Verification items for this drawing (mm, ordinates from the low corner). A direction names the side the tool comes from. Round coordinates to 2 decimals unless told otherwise and drop trailing zeros. Write each loop counter-clockwise with the first axis right and the second up, starting at its lowest first coordinate (ties: lowest second). Pieces come first, ordered by that corner, then holes. Notation, with made-up numbers: (-39, -31.5) -> (-17, -31.5) arc R27 ccw to (-17, -6.5) -> close; hole circle Ø2 at (64, 57.5). An arc over 180 degrees is marked (long way). One line per question, with ' | ' between items.
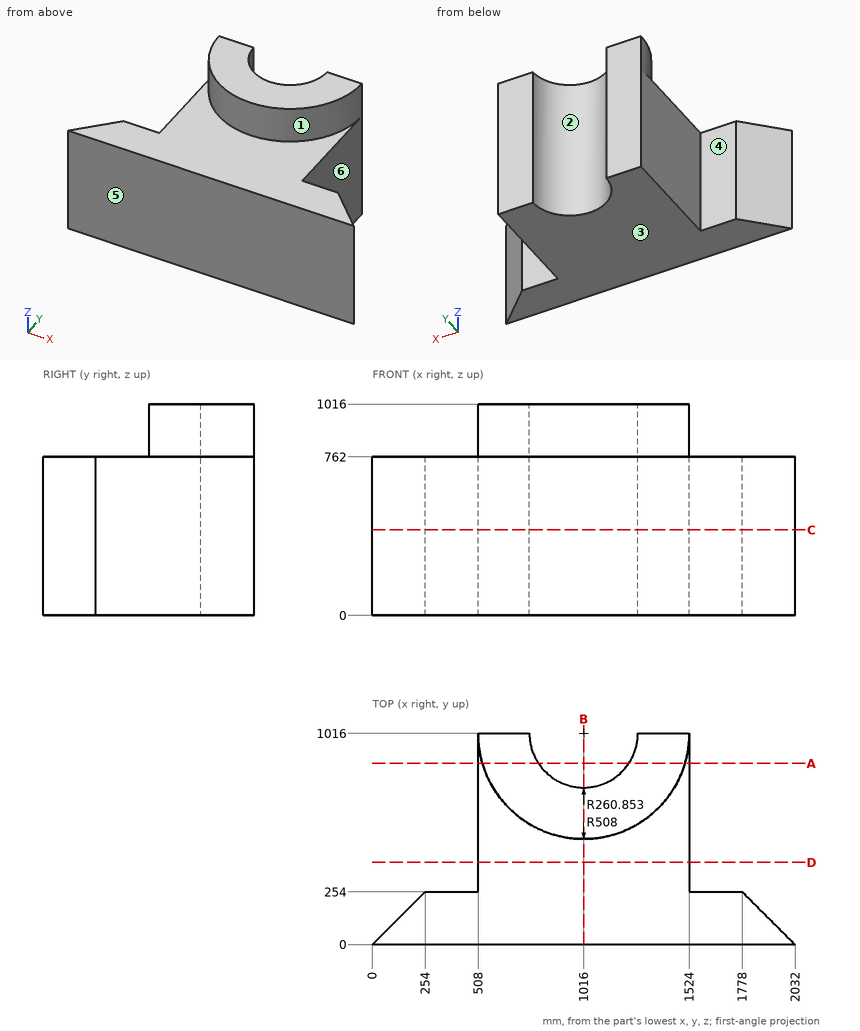
(1) Draft check along X on the marked faces 1, 2 and 3. Enter one of: +X half, -X half, draft (parallel to the pull), parting line (faces both ways), or undercut.
Resolved:
face 1: parting line | face 2: undercut | face 3: draft
(2) Sectioned sample at C-C on z = 411. Record the cut outline in (x, y), then the cut area to 3 significant figures.
Resolved:
outline: (0, 0) -> (2032, 0) -> (1778, 254) -> (1524, 254) -> (1524, 1016) -> (1276.85, 1016) arc R260.85 cw to (755.15, 1016) -> (508, 1016) -> (508, 254) -> (254, 254) -> close | area: 1,120,000 mm2
(3) Material ranges on line 1 (Y direction, x = 1621.5, z = 177); line 2 (X direction, y = 740.5, z = 738); line 3 (Z direction, x = 927, y = 256), recorded low to high.
Resolved:
line 1: y = 0 to 254 | line 2: x = 508 to 1524 | line 3: z = 0 to 762
(4) Access from +Z, -Z, +X, -X, +Y, -Y to the whole of each face (thin tool, end or side, straight path). Record for the marked faces 4, 5 and 6.
Resolved:
face 4: +Z, -Z, -X, +Y | face 5: +Z, -Z, +X, -X, -Y | face 6: +Z, -Z, +X, +Y
(5) Sectioned sample at B-B on x = 1016. Record the cut outline in (y, z), then the cut area to 3 significant figures.
Resolved:
outline: (0, 0) -> (755.15, 0) -> (755.15, 1016) -> (508, 1016) -> (508, 762) -> (0, 762) -> close | area: 638,000 mm2
(6) Sectioned sample at D-D on y = 395.5. Record the cut outline in (x, z), then the cut area to 3 significant figures.
Resolved:
outline: (508, 0) -> (1524, 0) -> (1524, 762) -> (508, 762) -> close | area: 774,000 mm2
(7) Go/stop test with flat-tipped pins: pin 1 (5 mm diameter, centred on y = 775, z = 816, fed in from -X); pin 2 (8 mm diameter, centred on y = 827.5, z = 498, fed in from +X); pin 3 (12 mm diameter, centred on y = 580.5, z = 855.5, fed in from +X). Record where each tip stops, or that it passes through.
Resolved:
pin 1: stops at x = 567.47 | pin 2: stops at x = 1524 | pin 3: stops at x = 1287.28
(8) Sectioned sample at A-A on y = 872. Record the cut outline in (x, z) (1 decimal).
Resolved:
outline: (508, 0) -> (798.5, 0) -> (798.5, 1016) -> (528.8, 1016) -> (528.8, 762) -> (508, 762) -> close; (1233.5, 0) -> (1524, 0) -> (1524, 762) -> (1503.2, 762) -> (1503.2, 1016) -> (1233.5, 1016) -> close
